Check sheet for the modelled part. Datum: model origin and axes. Units: mm. Face numbers are marked on the shaded views. A direction names the side the tool comes from. Round coordinates to 2 decimals unless told otherwise and drop trailing zeros. Loops run counter-clockwise (first coordinate to the right, second up) from the corner with the lowest first, then second, coordinate; pieces in that order, holes last. Notation, with made-up numbers: (-2, 77.25) -> (28, 77.25) arc R17 ccw to (28, 93.25) -> close; hole circle Ø5 at (79, -16). An arc over 180 degrees is marked (long way). One line per item, written item: value. Start each with the question number.
1. Cross-section at D-D on x = -37.5. Record the cut outline in (y, z).
2. Go/stop test with a flat-tipped pin: pin 1 (4 mm diameter, centred on x = -46, z = -10.5, fed in from -Y). Record where the tip stops, or that it passes through.
3. Material ranges on L1, parallel to X at y = -17.5, z = -43; L2, parallel to X at y = -19, z = -4.5; L3, parallel to Z at x = -59.5, y = -18.5, recorded low to high.
4. Cross-section at C-C on z = -41.5. Record the cut outline in (x, y).
5. Cross-section at A-A on y = -27. Record the cut outline in (x, z), then the cut area to 3 significant figures.
6. Release check for a two-part mould opening along X. For the marked faces 3, 4 and 5 record: +X half, -X half, draft (parallel to the pull), parting line (faces both ways), or undercut.
7. Cross-section at B-B on x = -11.5. Record the cut outline in (y, z), then the cut area to 3 significant figures.
8. Set-up check for the marked faces 1 and 2: record each of +Z, -Z, +X, -X, +Y, -Y from which the full face is reachable in a straight line by a thin tool's end or side.
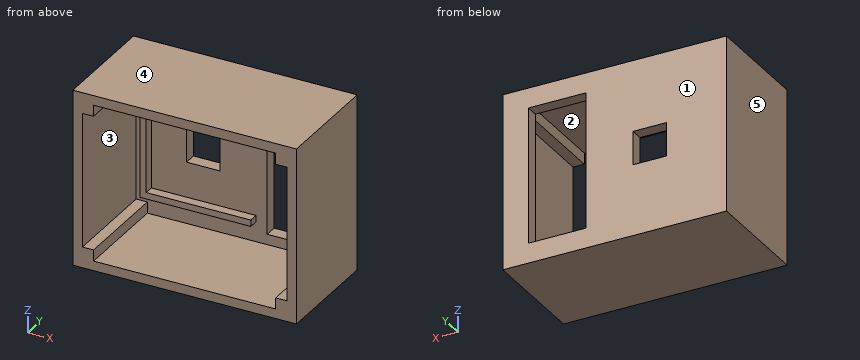
Autodesk Inventor part; units mm, degrees
ref_plane "YZ Plane" through (0, 0, 0) normal (1, 0, 0) x (0, 1, 0)
ref_plane "XZ Plane" through (0, 0, 0) normal (0, 1, 0) x (-1, 0, 0)
ref_plane "XY Plane" through (0, 0, 0) normal (0, 0, 1) x (1, 0, 0)
sketch "Sketch1" plane through (0, 0, 0) normal (0, 1, 0) x (-1, 0, 0)
  line L0 (0, 0) -> (70, 0)
  line L1 (70, 0) -> (70, -55)
  line L2 (70, -55) -> (0, -55)
  line L3 (0, -55) -> (0, 0)
  line L4 (51.25, -32.75) -> (40.75, -32.75)
  line L5 (40.75, -32.75) -> (40.75, -22.25)
  line L6 (40.75, -22.25) -> (51.25, -22.25)
  line L7 (51.25, -22.25) -> (51.25, -32.75)
  line L8 (26, -48.75) -> (8, -48.75)
  line L9 (8, -48.75) -> (8, -6.25)
  line L10 (8, -6.25) -> (26, -6.25)
  line L11 (26, -6.25) -> (26, -48.75)
  dimension "d0" = 70
  dimension "d1" = 55
  dimension "d2" = 10.5
  dimension "d3" = 10.5
  dimension "d4" = 18
  dimension "d5" = 42.5
  dimension "d6" = 6.25
  dimension "d7" = 22.25
  dimension "d8" = 8
  dimension "d9" = 18.75
extrude "Extrusion1" add sketch "Sketch1" along normal blind 4
sketch "Sketch2" plane through (0, 0, 0) normal (0, -1, 0) x (1, 0, 0)
  line L0 (0, 0) -> (0, -55)
  line L1 (-70, 0) -> (0, 0)
  line L2 (0, -55) -> (-70, -55)
  line L3 (-70, -55) -> (-70, 0)
  line L4 (-70, 0) -> (0, 0)
  line L5 (0, 0) -> (0, -55)
  line L6 (-3, -52) -> (-67, -52)
  line L7 (-67, -52) -> (-67, -3)
  line L8 (-67, -3) -> (-3, -3)
  line L9 (-3, -3) -> (-3, -52)
  line L10 (-29.5, -43.75) -> (-62.25, -43.75)
  line L11 (-62.25, -43.75) -> (-62.25, -11.25)
  line L12 (-62.25, -11.25) -> (-29.5, -11.25)
  line L13 (-40.75, -32.75) -> (-51.25, -32.75)
  line L14 (-51.25, -22.25) -> (-40.75, -22.25)
  line L15 (-51.25, -32.75) -> (-51.25, -22.25)
  line L16 (-40.75, -22.25) -> (-40.75, -32.75)
  line L17 (-29.5, -45.75) -> (-64.25, -45.75)
  line L18 (-64.25, -45.75) -> (-64.25, -9.25)
  line L19 (-64.25, -9.25) -> (-29.5, -9.25)
  line L20 (-29.5, -45.75) -> (-29.5, -43.75)
  line L21 (-29.5, -11.25) -> (-29.5, -9.25)
  dimension "d14" = 3
  dimension "d15" = 3
  dimension "d16" = 3
  dimension "d17" = 3
  dimension "d18" = 32.75
  dimension "d19" = 11
  dimension "d20" = 11
  dimension "d21" = 11
  dimension "d23" = 2
  dimension "d24" = 2
  dimension "d25" = 2
extrude "Extrusion2" add sketch "Sketch2" along normal blind 3 contours L20 L17 L18 L19 L21 L12 L11 L10
sketch "Sketch3" plane through (0, 0, 0) normal (0, -1, 0) x (1, 0, 0)
  line L0 (0, -55) -> (0, 0)
  line L1 (0, -55) -> (-70, -55)
  line L2 (-70, -55) -> (-70, 0)
  line L3 (-70, 0) -> (0, 0)
  line L4 (0, 0) -> (0, -55)
  line L5 (-3, -52) -> (-67, -52)
  line L6 (-67, -52) -> (-67, -3)
  line L7 (-67, -3) -> (-3, -3)
  line L8 (-3, -3) -> (-3, -52)
  dimension "d28" = 3
  dimension "d29" = 3
  dimension "d30" = 3
  dimension "d31" = 3
extrude "Extrusion3" add sketch "Sketch3" along normal blind 31
sketch "Sketch4" plane through (0, 0, 0) normal (0, -1, 0) x (1, 0, 0)
  line L0 (-3, -52) -> (-6.5, -52)
  line L1 (-6.5, -52) -> (-6.5, -48.5)
  line L2 (-6.5, -48.5) -> (-3, -48.5)
  line L3 (-3, -48.5) -> (-3, -52)
  line L4 (-3, -6.5116) -> (-3, -3.0116)
  line L5 (-67, -3) -> (-67, -52)
  line L6 (-67, -52) -> (-63.5, -52)
  line L7 (-63.5, -52) -> (-63.5, -48.5)
  line L8 (-63.5, -48.5) -> (-67, -48.5)
  line L9 (-67, -48.5) -> (-67, -52)
  line L10 (-67, -3) -> (-63.5, -3)
  line L11 (-63.5, -3) -> (-63.5, -6.5)
  line L12 (-63.5, -6.5) -> (-67, -6.5)
  line L13 (-67, -6.5) -> (-67, -3)
  line L14 (-3, -3) -> (-3, -52)
  line L15 (-3, -3) -> (-6.5, -3)
  line L16 (-6.5, -3) -> (-6.5, -6.5)
  line L17 (-6.5, -6.5) -> (-3, -6.5)
  line L18 (-3, -6.5) -> (-3, -3)
  point P0 (0, 0)
  dimension "d34" = 3.5
  dimension "d35" = 3.5
  dimension "d38" = 3.5
  dimension "d39" = 3.5
  dimension "d40" = 3.5
  dimension "d41" = 3.5
  dimension "d42" = 3.5
  dimension "d43" = 3.5
extrude "Extrusion4" add sketch "Sketch4" along normal blind 31
sketch "Sketch5" plane through (0, 4, 0) normal (1, 0, 0) x (0, 0, -1)
  line L0 (48.75, -16) -> (6.25, -16)
  line L1 (6.25, -16) -> (6.25, -35)
  line L2 (6.25, -35) -> (48.75, -35)
  line L3 (48.75, -35) -> (48.75, -16)
  line L4 (0, 0) -> (55, 0)
  line L5 (55, 0) -> (55, -35)
  point P0 (0, -4)
  dimension "d46" = 42.5
  dimension "d47" = 19
  dimension "d48" = 16
  dimension "d49" = 6.25
properties part number "test_camAndultra_sideprofiles"
Taken from the geometry:
1. outline: (-31, -55) -> (4, -55) -> (4, 0) -> (-31, 0) -> (-31, -3) -> (0, -3) -> (0, -9.25) -> (-3, -9.25) -> (-3, -11.25) -> (0, -11.25) -> (0, -43.75) -> (-3, -43.75) -> (-3, -45.75) -> (0, -45.75) -> (0, -52) -> (-31, -52) -> close
2. pin 1: stops at y = -3
3. L1: x = -70 to -67, -3 to 0
3. L2: x = -70 to -63.5, -6.5 to 0
3. L3: z = -55 to -52, -3 to 0
4. outline: (-70, -31) -> (-67, -31) -> (-67, 0) -> (-64.25, 0) -> (-64.25, -3) -> (-62.25, -3) -> (-62.25, 0) -> (-26, 0) -> (-26, 4) -> (-70, 4) -> close; (-8, 0) -> (-3, 0) -> (-3, -31) -> (0, -31) -> (0, 4) -> (-8, 4) -> close
5. outline: (-70, -55) -> (0, -55) -> (0, 0) -> (-70, 0) -> close; hole (-67, -48.5) -> (-63.5, -48.5) -> (-63.5, -52) -> (-6.5, -52) -> (-6.5, -48.5) -> (-3, -48.5) -> (-3, -6.5) -> (-6.5, -6.5) -> (-6.5, -3) -> (-63.5, -3) -> (-63.5, -6.5) -> (-67, -6.5) -> close
5. area: 763 mm2
6. face 3: undercut
6. face 4: draft
6. face 5: -X half
7. outline: (-31, -55) -> (4, -55) -> (4, -48.75) -> (0, -48.75) -> (0, -52) -> (-31, -52) -> close; (-31, -3) -> (0, -3) -> (0, -6.25) -> (4, -6.25) -> (4, 0) -> (-31, 0) -> close
7. area: 236 mm2
8. face 1: +Z, -Z, +X, -X, +Y
8. face 2: -Y
